CAD build for the part. Positions are in the model's coordinates, mm. Give positions to 0.01 mm unless a question says otherwise; leave off trailing zeros. Write each loop counter-clockwise with the first axis right and the second up, starting at its lowest first coordinate (ties: lowest second). Pieces come first, ordered by that corner, then holes. Notation, with made-up numbers: (70.25, 30.25) - (99.25, 30.25) arc R36 cw to (99.25, 64.25) - close; hole circle Ø1 at (28, 50). An arc over 180 degrees is marked (long way). Answer as a JSON object with one key per item and string values.
Solid Edge part; units mm, degrees
sketch "Sketch1" plane through (0, 0, 0) normal (0, 0, 1) x (1, 0, 0)
  line L0 (0, -121.1263) -> (180, -121.1263)
  line L1 (180, -121.1263) -> (180, 23.8737)
  line L2 (180, 23.8737) -> (0, 23.8737)
  line L3 (0, 23.8737) -> (0, -121.1263)
extrude "Protrusion1" add sketch "Sketch1" along normal blind 10
hole "Hole_3" at (141.5, 14.3737, 10) direction (0, 0, -1) diameter 6.6 end through all countersink diameter 12.6 countersink angle 90
hole "Hole1" at (141.5, -43.6263, 10) direction (0, 0, -1) diameter 6.6 end through all countersink diameter 12.6 countersink angle 90
hole "Hole2" at (38.5, -43.6263, 10) direction (0, 0, -1) diameter 6.6 end through all countersink diameter 12.6 countersink angle 90
hole "Hole3" at (38.5, 14.3737, 10) direction (0, 0, -1) diameter 6.6 end through all countersink diameter 12.6 countersink angle 90
hole "Hole_7" at (22, -14.6263, 0) direction (0, 0, 1) diameter 17.5 depth 50.8 countersink diameter 31 countersink angle 90
hole "Hole4" at (22, -87.6263, 0) direction (0, 0, 1) diameter 17.5 depth 50.8 countersink diameter 31 countersink angle 90
hole "Hole5" at (158, -87.6263, 0) direction (0, 0, 1) diameter 17.5 depth 50.8 countersink diameter 31 countersink angle 90
hole "Hole6" at (158, -14.6263, 0) direction (0, 0, 1) diameter 17.5 depth 50.8 countersink diameter 31 countersink angle 90
properties material "Aluminum, 6061-T6"
(1) Pull direction X, two halves, no side cores. Call faces 1 (the face through (138.28, -42.91, 3.55)), 2 (the face through (180, -50, 5)), 3 (the face through (89, -121.126, 5)): pulls with the +X half, pulls with the -X half, needs draft (parallel to the pull), parting line crosses it, or undercut.
Answer key:
{"face 1": "undercut", "face 2": "pulls with the +X half", "face 3": "needs draft"}
(2) Flat gauge pins, fed straight in: P1, Ø20, axis at x = 158, y = -14.63, coming from the -Z side; P2, Ø6, axis at x = 141.5, y = 14.37, coming from the -Z side; P3, Ø7.5, axis at x = 38.5, y = 14.37, coming from the +Z side. Where does each tip first touch, or does it go through?
Answer key:
{"P1": "stops at z = 5.5", "P2": "passes through", "P3": "stops at z = 7.45"}
(3) Saw through at B-B, the plane z = 5. State how many separate pieces and enclosed holes the cut face has, and give its area (3 significant figures).
Answer key:
{"separate pieces": "1", "enclosed holes": "8", "area": "24,600 mm²"}
(4) Saw through at A-A, the plane x = 22. Give the cut face in (y, z), and give its area (3 significant figures).
Answer key:
{"outline": "(-121.13, 0) - (-103.13, 0) - (-96.38, 6.75) - (-96.38, 10) - (-121.13, 10) - close; (-78.88, 6.75) - (-72.13, 0) - (-30.13, 0) - (-23.38, 6.75) - (-23.38, 10) - (-78.88, 10) - close; (-5.88, 6.75) - (0.87, 0) - (23.87, 0) - (23.87, 10) - (-5.88, 10) - close", "area": "1,010 mm²"}
(5) Probe L1, parallel to Y at x = 22, z = 8.15; L2, parallel to Y at x = 38.5, z = 1; L3, parallel to X at y = -7, z = 7.75. List the from-to ranges inside material, lowest first. Write a range as [from, to].
Answer key:
{"L1": "y = [-121.13, -96.38], [-78.88, -23.38], [-5.88, 23.87]", "L2": "y = [-121.13, -46.93], [-40.33, 11.07], [17.67, 23.87]", "L3": "x = [0, 17.71], [26.29, 153.71], [162.29, 180]"}
